```python
from build123d import *

# Parameters (mm, degrees)
SKETCH1_R           = 3.5
BOSS_EXTRUDE2_DEPTH = 2
SKETCH2_R           = 3.5
BOSS_EXTRUDE3_DEPTH = 3


with BuildPart() as part:
    # Sketch1 → Boss-Extrude2 (new body)
    with BuildSketch(Plane.XY):
        with BuildLine():
            ThreePointArc((31.828129573, 31.962855422), (26.925185535, 34.12264134), (21.93108129, 32.182935631))
            Line((21.93108129, 32.182935631), (-32.990473375, -20.349176769))
            ThreePointArc((-32.990473375, -20.349176769), (-35.150259292, -25.252120806), (-33.210553583, -30.246225051))
            Line((-33.210553583, -30.246225051), (-31.828129573, -31.691529121))
            ThreePointArc((-31.828129573, -31.691529121), (-26.925185535, -33.851315038), (-21.93108129, -31.91160933))
            Line((-21.93108129, -31.91160933), (32.990473375, 20.62050307))
            ThreePointArc((32.990473375, 20.62050307), (35.150259292, 25.523447107), (33.210553583, 30.517551352))
            Line((33.210553583, 30.517551352), (31.828129573, 31.962855422))
        make_face()
        with Locations((26.738125297, 25.710507345)):
            Circle(SKETCH1_R, mode=Mode.SUBTRACT)
    extrude(amount=BOSS_EXTRUDE2_DEPTH)

    # Sketch2 → Boss-Extrude3 (add)
    with BuildSketch(Plane.XY.offset(2)):
        with Locations((-26.738125297, -25.439181044)):
            Circle(SKETCH2_R)
    extrude(amount=BOSS_EXTRUDE3_DEPTH)


solid = part.part
```
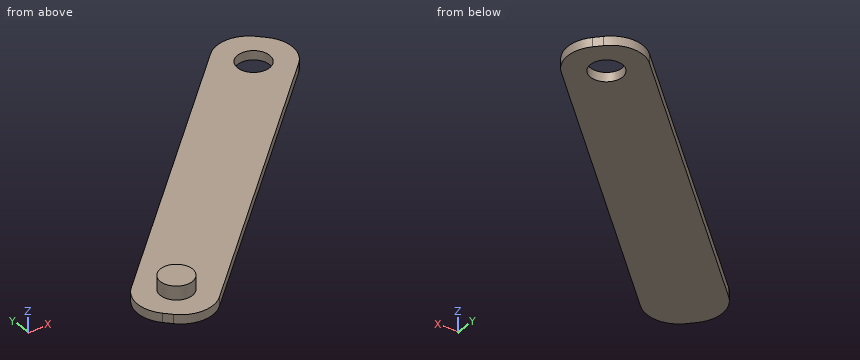
Design review of the part built by this model. Coordinates are the model's own, in mm. Give positions to 0.01 mm unless a question says otherwise; leave off trailing zeros. Write each loop counter-clockwise with the first axis right and the second up, starting at its lowest first coordinate (ties: lowest second). Pieces come first, ordered by that corner, then holes. Notation, with made-up numbers: (7, 86) - (33, 86) arc R21 ccw to (33, 107) - close; hole circle Ø4 at (88, 84). An arc over 180 degrees is marked (long way). Return JSON: item names as keys, results as strings. Group by question number.
(1) We need section C-C, the plane y = -5.5. Give the boundary of the cut face in (x, z), then the cut area to 3 significant figures.
(2) Insertion check: pin 1 (8 mm diameter, centred on x = 14, y = 7.5, fed in from +Z); pin 2 (2 mm diameter, centred on y = -11.5, z = 1, fed in from -X); pin 3 (5 mm diameter, centred on x = -23.5, y = -12, fed in from -Z); pin 4 (3 mm diameter, centred on x = 21, z = 3, fed in from +Y). Each pin has a flat end and moves straight along its axis. Give the tip position at first contact, or say it passes through.
(3) We need section B-B, the plane z = 0.8. Give the boundary of the cut face in (x, y).
(4) We need section D-D, the plane x = -9. Give the boundary of the cut face in (y, z), then the cut area to 3 significant figures.
(5) We need section A-A, the plane x = 26. Give the boundary of the cut face in (y, z).
(6) To check wall thickness, follow probe 1 along Z at (x, y) = (0.5, 7); probe 2 along Y at (x, z) = (-27, 2.6); probe 3 along Y at (x, z) = (17.5, 0.35). State the ranges of each line that lie inside material, in increasing order.
Reported:
{
 "1": {"outline": "(-17.47, 0) - (5.68, 0) - (5.68, 2) - (-17.47, 2) - close", "area": "46.3 mm2"},
 "2": {"pin 1": "stops at z = 2", "pin 2": "stops at x = -24.78", "pin 3": "stops at z = 0", "pin 4": "stops at y = 32.36"},
 "3": {"outline": "(-33.21, -30.25) - (-31.83, -31.69) arc R7 ccw to (-21.93, -31.91) - (32.99, 20.62) arc R7 ccw to (33.21, 30.52) - (31.83, 31.96) arc R7 ccw to (21.93, 32.18) - (-32.99, -20.35) arc R7 ccw to start; hole circle Ø7 at (26.74, 25.71)"},
 "4": {"outline": "(-19.54, 0) - (2.6, 0) - (2.6, 2) - (-19.54, 2) - close", "area": "44.3 mm2"},
 "5": {"outline": "(13.93, 0) - (22.29, 0) - (22.29, 2) - (13.93, 2) - close; (29.13, 0) - (34.08, 0) - (34.08, 2) - (29.13, 2) - close"},
 "6": {"probe 1": "z = 0 to 2", "probe 2": "y = -28.93 to -21.95", "probe 3": "y = 5.8 to 27.94"}
}
